Work out the finished part from the listing and answer in its coordinate system (mm). Face numbers are marked on the shaded views. A direction names the side the tool comes from. Round coordinates to 2 decimals unless told otherwise and drop trailing zeros. Loops run counter-clockwise (first coordinate to the right, second up) from the corner with the lowest first, then second, coordinate; pieces in that order, holes last. Notation, with made-up numbers: (3, 77) -> (43, 77) arc R17 cw to (43, 105) -> close; hole circle Ø9 at (61, 59.5). An arc over 180 degrees is marked (long way). Use one line per item in the form item = value.
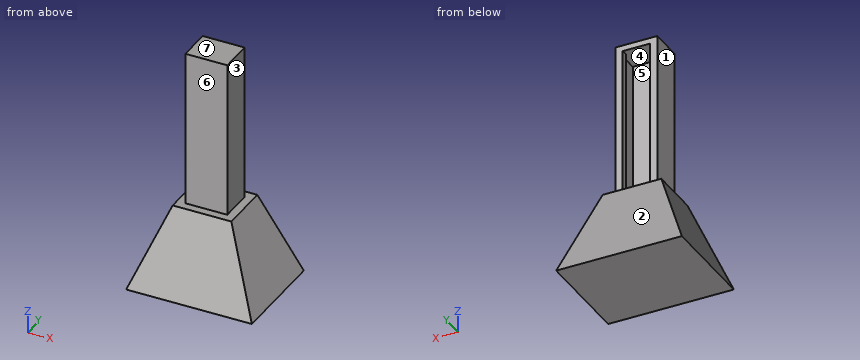
```python
from build123d import *

# Parameters (mm, degrees)
SKETCH2_W           = 750
SKETCH2_H           = 600
BOSS_EXTRUDE1_DEPTH = 500
CUT_EXTRUDE2_DEPTH  = 867.386172558
CUT_EXTRUDE3_DEPTH  = 951
BOSS_EXTRUDE2_DEPTH = 900
SKETCH6_W           = 35
SKETCH6_H           = 200
BOSS_EXTRUDE3_DEPTH = 250


with BuildPart() as part:
    # Sketch2 → Boss-Extrude1 (new body)
    with BuildSketch(Plane.XY):
        Rectangle(SKETCH2_W, SKETCH2_H)
    extrude(amount=-BOSS_EXTRUDE1_DEPTH)

    # Sketch3 → Cut-Extrude2 (cut, through all)
    with BuildSketch(Plane.XZ.offset(300)):
        Polygon((-375, -500), (-375, 0), (-175, 0), align=None)
        Polygon((375, 0), (175, 0), (375, -500), align=None)
    extrude(amount=-CUT_EXTRUDE2_DEPTH, mode=Mode.SUBTRACT)

    # Sketch4 → Cut-Extrude3 (cut, through all)
    with BuildSketch(Plane(origin=(375, 0, 0), x_dir=(0, 0, -1), z_dir=(1, 0, 0))):
        Polygon((500, -300), (0, -300), (0, -150), align=None)
        Polygon((0, 300), (0, 150), (500, 300), align=None)
    extrude(amount=-CUT_EXTRUDE3_DEPTH, mode=Mode.SUBTRACT)

    # Sketch5 → Boss-Extrude2 (add)
    with BuildSketch(Plane.XY):
        Polygon((-81.25, 65), (-81.25, 100), (-125, 100), (-125, -100), (-81.25, -100), (81.25, -100), (125, -100), (125, 100), (81.25, 100), (81.25, 65), (106.25, 65), (106.25, -65), (81.25, -65), (-81.25, -65), (-106.25, -65), (-106.25, 65), align=None)
    extrude(amount=BOSS_EXTRUDE2_DEPTH)

    # Sketch6 → Boss-Extrude3 (add)
    with BuildSketch(Plane(origin=(125, 0, 0), x_dir=(0, 0, -1), z_dir=(1, 0, 0))):
        with Locations((-917.5, 0)):
            Rectangle(SKETCH6_W, SKETCH6_H)
    extrude(amount=-BOSS_EXTRUDE3_DEPTH)


solid = part.part
```
(1) For the marked faces 1, 2 and 3, determine the directions among +Z, -Z, +X, -X, +Y, -Y from which every point of the face is accessible in a straight line to the end or side of a thin tool.
Completed:
face_1 = +Z, -X, +Y, -Y
face_2 = +Z, +X, -X, +Y
face_3 = +Z, +X, +Y, -Y
(2) Find section A-A, the plane y = -30. Write down the section's boundary in (x, z).
Completed:
outline = (-375, -500) -> (375, -500) -> (175, 0) -> (125, 0) -> (125, 935) -> (-125, 935) -> (-125, 0) -> (-175, 0) -> close; hole (-106.25, 0) -> (106.25, 0) -> (106.25, 900) -> (-106.25, 900) -> close
(3) Find section B-B, the plane z = 711. Write down the section's boundary in (x, y).
Completed:
outline = (-125, -100) -> (125, -100) -> (125, 100) -> (81.25, 100) -> (81.25, 65) -> (106.25, 65) -> (106.25, -65) -> (-106.25, -65) -> (-106.25, 65) -> (-81.25, 65) -> (-81.25, 100) -> (-125, 100) -> close
(4) Find section C-C, the plane x = -14. Write down the section's boundary in (y, z).
Completed:
outline = (-300, -500) -> (300, -500) -> (150, 0) -> (-65, 0) -> (-65, 900) -> (100, 900) -> (100, 935) -> (-100, 935) -> (-100, 0) -> (-150, 0) -> close
(5) Given P1, Ø12.5, axis at x = 91, z = 229.5, coming from the -Y side; P2, Ø4, axis at y = 77.5, z = 364.5, coming from the +X side; P3, Ø1, axis at x = 50, y = -141.5, coming from the +Z side, each flat-ended and moving along its own axis, determine where each tip first touches the part or whether it passes through.
Completed:
P1 = -100
P2 = 125
P3 = 0
(6) Find section D-D, the plane y = -237. Write down the section's boundary in (x, z).
Completed:
outline = (-375, -500) -> (375, -500) -> (291, -290) -> (-291, -290) -> close
(7) Consider L1, parallel to X at y = 57.5, z = 406; L2, parallel to X at y = 80, z = 146; L3, parallel to Z at x = 106, y = 42.5. Determine where each line is inside the solid, lowest interval first.
Completed:
L1 = -125 to -106.25, 106.25 to 125
L2 = -125 to -81.25, 81.25 to 125
L3 = -500 to 0, 900 to 935
(8) For a pull along Z with two mould halves and no side action, classify the marked faces 4, 5, 6 and 7 as +Z half, -Z half, draft (parallel to the pull), parting line (faces both ways), or undercut.
Completed:
face_4 = undercut
face_5 = undercut
face_6 = draft
face_7 = +Z half
